Autodesk Fusion 360 part; units mm, degrees
sketch "Sketch1" plane through (0, 0, 0) normal (0, 0, 1) x (1, 0, 0)
  line L0 (12.5, -42) -> (-12.5, -42)
  line L1 (-12.5, -42) -> (-12.5, 42)
  line L2 (-12.5, 42) -> (12.5, 42)
  line L3 (12.5, 42) -> (12.5, -42)
  line L4 (12.5, -42) -> (-12.5, 42) construction
  line L5 (-12.5, -42) -> (12.5, 42) construction
  line L6 (10, -20) -> (-10, -20)
  line L7 (-10, -20) -> (-10, 20)
  line L8 (-10, 20) -> (10, 20)
  line L9 (10, 20) -> (10, -20)
  line L10 (10, -20) -> (-10, 20) construction
  line L11 (-10, -20) -> (10, 20) construction
  circle A0 centre (5, -24) radius 2.5
  circle A1 centre (-5, -24) radius 2.5
  line L12 (0, 0) -> (5, 0) construction
  circle A2 centre (5, 24) radius 2.5
  circle A3 centre (-5, 24) radius 2.5
  circle A4 centre (6.5, 35) radius 2.5
  circle A5 centre (-6.5, 35) radius 2.5
  circle A6 centre (6.5, -35) radius 2.5
  circle A7 centre (-6.5, -35) radius 2.5
  dimension "d1" = 84
  dimension "d2" = 25
  dimension "d3" = 40
  dimension "d4" = 20
  dimension "d5" = 5
  dimension "d6" = 5
  dimension "d7" = 18
  dimension "d8" = 18
  dimension "d9" = 5
  dimension "d10" = 10
  dimension "d11" = 5
  dimension "d12" = 5
  dimension "d13" = 6
  dimension "d14" = 7
  dimension "d15" = 13
  dimension "d16" = 7
extrude "Extrude1" add sketch "Sketch1" along normal blind 9
Read the model definition and answer for the solid it produces. Units are mm, in the model's axes. A direction names the side the tool comes from. Coordinates: 2 decimals unless noted, no trailing zeros. Write each loop counter-clockwise with the first axis right and the second up, starting at its lowest first coordinate (ties: lowest second). Pieces come first, ordered by that corner, then holes. Notation, with made-up numbers: (10, 9.5) -> (43, 9.5) arc R19 ccw to (43, 18.5) -> close; hole circle Ø2 at (78.5, -2.5). An arc over 180 degrees is marked (long way). Return JSON: item names as keys, results as strings.
1. A cutting plane is placed at A-A (x = -6.5). Determine the outline of the cut face in (y, z), and give its area (3 significant figures).
Found:
{"outline": "(-42, 0) -> (-37.5, 0) -> (-37.5, 9) -> (-42, 9) -> close; (-32.5, 0) -> (-26, 0) -> (-26, 9) -> (-32.5, 9) -> close; (-22, 0) -> (-20, 0) -> (-20, 9) -> (-22, 9) -> close; (20, 0) -> (22, 0) -> (22, 9) -> (20, 9) -> close; (26, 0) -> (32.5, 0) -> (32.5, 9) -> (26, 9) -> close; (37.5, 0) -> (42, 0) -> (42, 9) -> (37.5, 9) -> close", "area": "234 mm2"}
2. Determine the mould class of faces 3 (the face through (-10, 0, 4)), 4 (the face through (-12.5, -1, 4)), 5 (the face through (0, -42, 4)) for opening direction Y: pulls with the +Y half, pulls with the -Y half, needs draft (parallel to the pull), parting line crosses it, or undercut.
Found:
{"face 3": "undercut", "face 4": "needs draft", "face 5": "pulls with the -Y half"}
3. A cutting plane is placed at C-C (y = -15.5). Determine the outline of the cut face in (x, z), and give its area (3 significant figures).
Found:
{"outline": "(-12.5, 0) -> (-10, 0) -> (-10, 9) -> (-12.5, 9) -> close; (10, 0) -> (12.5, 0) -> (12.5, 9) -> (10, 9) -> close", "area": "45.0 mm2"}
4. Find the intervals of material crossed by line 1 along X through (y, z) = (-17, 8.5); line 2 along X through (y, z) = (23, 5.25); line 3 along Y through (x, z) = (-5.75, 3.25), in increasing order. Write a range as from..to.
Found:
{"line 1": "-12.5..-10, 10..12.5", "line 2": "-12.5..-7.29, -2.71..2.71, 7.29..12.5", "line 3": "-42..-37.38, -32.62..-26.38, -21.62..-20, 20..21.62, 26.38..32.62, 37.38..42"}
5. A cutting plane is placed at D-D (x = -1.75). Determine the outline of the cut face in (y, z), and give its area (3 significant figures).
Found:
{"outline": "(-42, 0) -> (-20, 0) -> (-20, 9) -> (-42, 9) -> close; (20, 0) -> (42, 0) -> (42, 9) -> (20, 9) -> close", "area": "396 mm2"}
6. A cutting plane is placed at B-B (y = -35). Determine the outline of the cut face in (x, z), and give its area (3 significant figures).
Found:
{"outline": "(-12.5, 0) -> (-9, 0) -> (-9, 9) -> (-12.5, 9) -> close; (-4, 0) -> (4, 0) -> (4, 9) -> (-4, 9) -> close; (9, 0) -> (12.5, 0) -> (12.5, 9) -> (9, 9) -> close", "area": "135 mm2"}
7. This flat-tipped pin is pushed along its axis until it touches: P1, Ø1.5, axis at x = -0.5, y = -20.5, coming from the -Z side. Where does it stop, or does it pass through?
Found:
{"P1": "z = 0"}
8. A tool of negligible diameter and unlimited length cuts with its end or side. For faces 1 (the face through (0, 20, 4)), 2 (the face through (0, 42, 4)), from which of +Z, -Z, +X, -X, +Y, -Y can it reach the whole face along a straight path? Write none if from no direction.
Found:
{"face 1": "+Z, -Z", "face 2": "+Z, -Z, +X, -X, +Y"}
